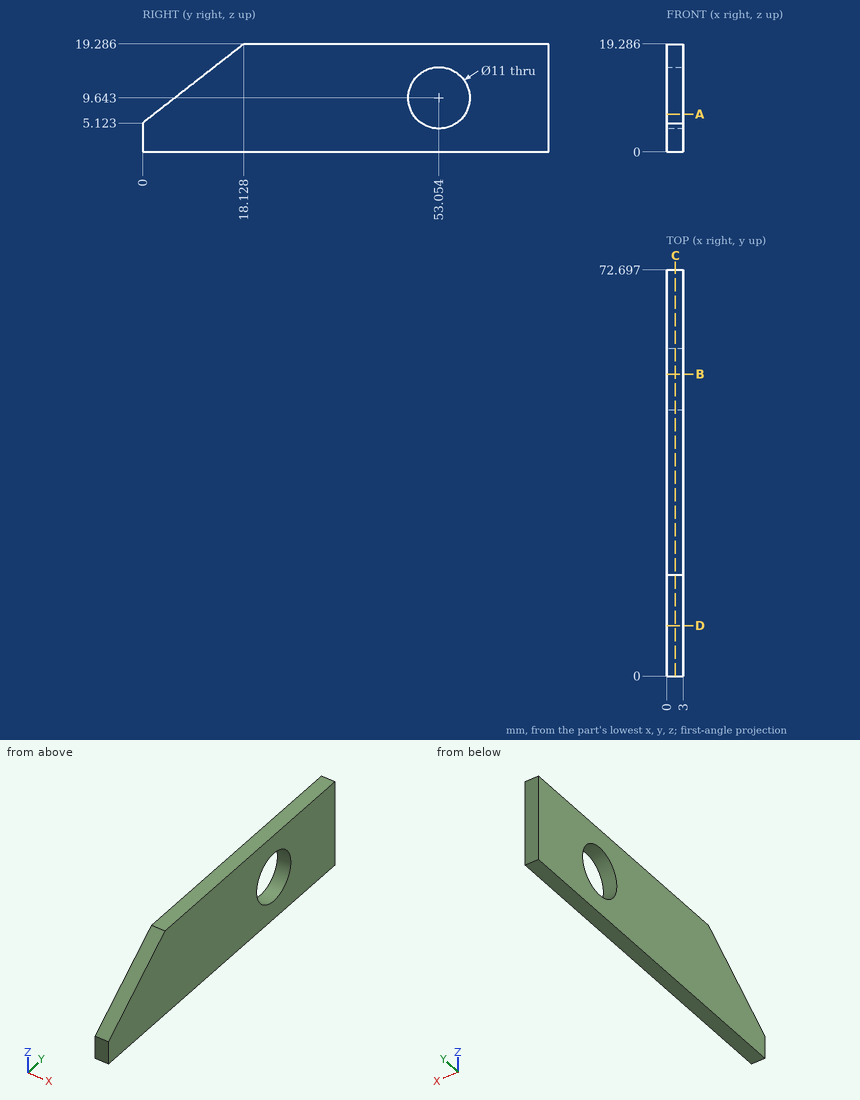
Verification items for this drawing (mm, ordinates from the low corner). Coordinates: 2 decimals unless noted, no trailing zeros. Order: outer loops, then holes, each group sorted by start corner. A loop starts at its lowest first (then second) coordinate and runs counter-clockwise, first axis right, second up. Notation, with made-up numbers: (-6, 68) - (25, 68) arc R14 cw to (25, 82) - close; hole circle Ø11 at (55, -4). An arc over 180 degrees is marked (long way). Use one line per item in the form item = value.
1. Section check A-A (z = 6.75). Record the boundary of the cut face in (x, y).
Here are the results:
outline = (0, 2.08) - (3, 2.08) - (3, 48.38) - (0, 48.38) - close; (0, 57.73) - (3, 57.73) - (3, 72.7) - (0, 72.7) - close
2. Section check C-C (x = 1.55). Record the boundary of the cut face in (y, z) (1 decimal), then the cut area to 3 significant figures.
Here are the results:
outline = (0, 0) - (72.7, 0) - (72.7, 19.3) - (18.1, 19.3) - (0, 5.1) - close; hole circle Ø11 at (53.1, 9.6)
area = 1,180 mm²
3. Section check D-D (y = 9). Record the boundary of the cut face in (x, z) (1 decimal).
Here are the results:
outline = (0, 0) - (3, 0) - (3, 12.2) - (0, 12.2) - close
4. Section check B-B (y = 54). Record the boundary of the cut face in (x, z) (1 decimal).
Here are the results:
outline = (0, 0) - (3, 0) - (3, 4.2) - (0, 4.2) - close; (0, 15.1) - (3, 15.1) - (3, 19.3) - (0, 19.3) - close
5. Scan lines: line 1 (Y direction, x = 0.3, z = 12.25) (1 decimal); line 2 (Y direction, x = 1.7, z = 5.25) (1 decimal); line 3 (Z direction, x = 0.1, y = 51.5) (1 decimal). Record each from-to range of solid material in increasing order.
Here are the results:
line_1 = 9.1 to 48.2, 57.9 to 72.7
line_2 = 0.2 to 49.7, 56.4 to 72.7
line_3 = 0 to 4.4, 14.9 to 19.3
